Check sheet for the modelled part. Datum: model origin and axes. Units: mm. Give positions to 0.01 mm unless a question says otherwise; leave off trailing zeros. Order: outer loops, then holes, each group sorted by start corner. A loop starts at its lowest first (then second) coordinate and runs counter-clockwise, first axis right, second up. Notation, with made-up numbers: M 74.5,76 L 122.5,76 A13 cw 122.5,87 Z; hole C 61.25,-27 d7. An arc over 180 degrees is marked long. Return JSON: item names as keys, results as strings. Group by question number.
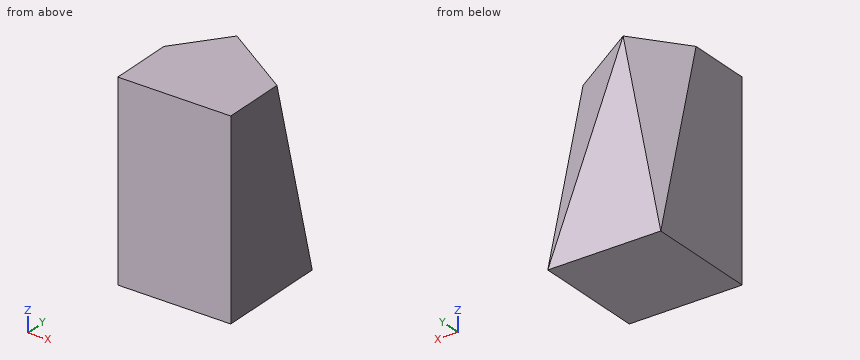
from build123d import *

# Parameters (mm, degrees)
SKETCH2_W           = 30
SKETCH2_H           = 51
BOSS_EXTRUDE1_DEPTH = 30


with BuildPart() as part:
    # Sketch2 → Boss-Extrude1 (new body)
    with BuildSketch(Plane(origin=(0, 0, 0), x_dir=(1, 0, 0), z_dir=(0, 1, 0))):
        with Locations((15, 25.5)):
            Rectangle(SKETCH2_W, SKETCH2_H)
    extrude(amount=BOSS_EXTRUDE1_DEPTH)

    # SurfaceCut2
    split(bisect_by=Plane(origin=(15.949847794, 24.538227375, 6.254842272), x_dir=(0.8461451498623624, -0.5164387356010117, -0.1316412463296696), z_dir=(0.5329525169885216, 0.8199269492131106, 0.20900098705432213)), keep=Keep.BOTTOM)

    # SurfaceCut3
    split(bisect_by=Plane(origin=(-8.02185135, 6.170654885, 1.572912029), x_dir=(-0.1217254970638359, 0.09363499774141223, -0.9881373338572569), z_dir=(0.7832213553451228, -0.6024779656500949, -0.15357281477355358)), keep=Keep.TOP)


solid = part.part
1) Material ranges on line 1 along Y through (x, z) = (6, -11.5); line 2 along X through (y, z) = (25.5, -7); line 3 along Y through (x, z) = (25.5, -20), recorded low to high.
2) Sectioned sample at B-B on z = -32. Record the boundary of the cut face in (x, y).
3) Sectioned sample at D-D on x = 2.5. Record the boundary of the cut face in (y, z).
4) Sectioned sample at A-A on x = 20. Record the boundary of the cut face in (y, z), then the cut area to 3 significant figures.
5) Sectioned sample at C-C on y = 24.5. Record the boundary of the cut face in (x, z), then the cut area to 3 significant figures.
Reply:
{
 "1": {"line 1": "0 to 27.73", "line 2": "5.17 to 19.67", "line 3": "0 to 25.02"},
 "2": {"outline": "M 0,0 L 30,0 L 30,25.16 L 22.55,30 L 3.73,30 L 0,25.16 Z"},
 "3": {"outline": "M 0,-51 L 30,-51 L 30,-38.25 L 20.25,0 L 0,0 Z"},
 "4": {"outline": "M 0,-51 L 30,-51 L 30,-25.5 L 23.5,0 L 0,0 Z", "area": "1,450 mm^2"},
 "5": {"outline": "M 0,-51 L 30,-51 L 30,-29.42 L 18.46,0 L 5.77,0 L 0,-29.42 Z", "area": "1,280 mm^2"}
}
